Can you work these out from the model? Positions are in its coordinate system, mm. A direction names the side the tool comes from. Coordinates: 2 decimals unless noted, no trailing zeros. Order: outer loops, then holes, each group sorted by start corner. A loop starts at its lowest first (then second) coordinate and runs counter-clockwise, first axis right, second up. Notation, with made-up numbers: (-5, 43) -> (15, 43) arc R26 ccw to (15, 63) -> close; hole circle Ø11 at (-13.75, 67.5). An arc over 180 degrees is marked (long way). Return JSON: item names as keys, results as strings. Group by question number.
1) If we section it at A-A, the plane z = 0: State how many separate pieces and enclosed holes the cut face has, then the cut area to 3 significant figures.
2) If I drill on probe 1 along X at (y, z) = (5, -3); probe 2 along Y at (x, z) = (19.5, -0.5); probe 3 along X at (y, z) = (12, -4.25), over which ranges is the centre line in solid material (lowest first)? Write a range as from..to.
3) Thinking about a two-plate mould opening in X: for faces 6 (the flat face through (0, 0, 0)), 7 (the flat face through (-26.75, 7, 0)), 8 (the cylindrical face through (28.449, 6.409, -4.715)), which applies, +X half, -X half, draft (parallel to the pull), parting line (faces both ways), or undercut?
4) For faces 1 (the cylindrical face through (-27.051, 7.577, -4.715)), 2 (the cylindrical face through (-27.051, 7.07, 4.715)), 3 (the cylindrical face through (-28.465, 12.699, -0.563)), 4 (the cylindrical face through (-27.051, 12.715, -0.563)), 5 (the flat face through (28.75, 6, 0)), which set-ups out of +Z, -Z, +X, -X, +Y, -Y let a thin tool reach every point of the face, with its end or its side?
5) If we section it at B-B, the plane x = 3.5: Please give me the cut outline in (y, z).
6) For pin 1 (6 mm diameter, centred on x = 6.5, z = -2.5, fed in from +Y), with a flat end and sliding along its axis, tell me the tip position at first contact or that it passes through.
from build123d import *

# Parameters (mm, degrees)
SKETCH1_W           = 57.5
SKETCH1_H           = 10
BOSS_EXTRUDE1_DEPTH = 3
SKETCH2_W           = 2
SKETCH2_H           = 10
BOSS_EXTRUDE2_DEPTH = 10
SKETCH3_R           = 1.5
CUT_EXTRUDE1_DEPTH  = 60.162910679
FILLET1_R           = 1


with BuildPart() as part:
    # Sketch1 → Boss-Extrude1 (new body)
    with BuildSketch(Plane(origin=(0, 0, 0), x_dir=(1, 0, 0), z_dir=(0, 1, 0))):
        Rectangle(SKETCH1_W, SKETCH1_H)
    extrude(amount=BOSS_EXTRUDE1_DEPTH)

    # Sketch2 → Boss-Extrude2 (add)
    with BuildSketch(Plane(origin=(0, 3, 0), x_dir=(1, 0, 0), z_dir=(0, 1, 0))):
        with Locations((-27.75, 0)):
            Rectangle(SKETCH2_W, SKETCH2_H)
        with Locations((27.75, 0)):
            Rectangle(SKETCH2_W, SKETCH2_H)
    extrude(amount=BOSS_EXTRUDE2_DEPTH)

    # Sketch3 → Cut-Extrude1 (cut, through all)
    with BuildSketch(Plane.ZY.offset(28.75)):
        with Locations((0, 9.287412426)):
            Circle(SKETCH3_R)
    extrude(amount=-CUT_EXTRUDE1_DEPTH, mode=Mode.SUBTRACT)

    # Fillet1
    fillet1_edges = [part.edges().sort_by_distance(p)[0] for p in [
        (0, 3, 5),
        (-26.75, 8, 5),
        (-26.75, 8, -5),
        (-28.75, 13, 0),
        (-27.75, 13, 5),
        (-26.75, 13, 0),
        (0, 3, -5),
        (26.75, 8, -5),
        (26.75, 8, 5),
        (28.75, 13, 0),
        (26.75, 13, 0),
        (27.75, 13, 5),
        (0, 0, 5),
        (-28.75, 0, 0),
        (0, 0, -5),
        (28.75, 6.5, 5),
        (-28.75, 6.5, 5),
        (-28.75, 6.5, -5),
        (28.75, 6.5, -5),
    ]]
    fillet(fillet1_edges, radius=FILLET1_R - 0.0001)  # a hair under: the kernel refuses the full size


solid = part.part
Result sheet:
{
 "1": {"separate pieces": "3", "enclosed holes": "0", "area": "199 mm2"},
 "2": {"probe 1": "x = -28.75..-26.75, 26.75..28.75", "probe 2": "y = 0..3", "probe 3": "x = -28.72..-26.78, 26.78..28.72"},
 "3": {"face 6": "draft", "face 7": "undercut", "face 8": "+X half"},
 "4": {"face 1": "-Z, +Y", "face 2": "+Z, +Y", "face 3": "+Z, -Z, -X, +Y", "face 4": "+Z, -Z, +Y", "face 5": "+Z, -Z, +X, +Y, -Y"},
 "5": {"outline": "(0, -4) arc R1 ccw to (1, -5) -> (2, -5) arc R1 ccw to (3, -4) -> (3, 4) arc R1 ccw to (2, 5) -> (1, 5) arc R1 ccw to (0, 4) -> close"},
 "6": {"pin 1": "stops at y = 3"}
}
